```python
from build123d import *

# Parameters (mm, degrees)
SKETCH_1_W      = 27.85
SKETCH_1_H      = 27.85
SKETCH_1_R      = 1.25
SKETCH_1_R_2    = 6.5
EXTRUDE_1_DEPTH = 7
SKETCH_1_5_R    = 11
SKETCH_1_5_R_2  = 6.5
EXTRUDE_3_DEPTH = 9
CHAMFER_2_SIZE  = 0.4
CHAMFER_3_SIZE  = 0.2
FILLET_1_R      = 2


with BuildPart() as part:
    # Эскиз1 → Бобышка-Вытянуть1 (new body)
    with BuildSketch(Plane(origin=(0, 0, 0), x_dir=(1, 0, 0), z_dir=(0, 1, 0))):
        Rectangle(SKETCH_1_W, SKETCH_1_H)
        with Locations((-11.5, 11.5)):
            Circle(SKETCH_1_R, mode=Mode.SUBTRACT)
        with Locations((11.5, 11.5)):
            Circle(SKETCH_1_R, mode=Mode.SUBTRACT)
        with Locations((-11.5, -11.5)):
            Circle(SKETCH_1_R, mode=Mode.SUBTRACT)
        with Locations((11.5, -11.5)):
            Circle(SKETCH_1_R, mode=Mode.SUBTRACT)
        Circle(SKETCH_1_R_2, mode=Mode.SUBTRACT)
    extrude(amount=EXTRUDE_1_DEPTH)

    # Эскиз1<5> → Бобышка-Вытянуть3 (add)
    with BuildSketch(Plane(origin=(0, 0, 0), x_dir=(1, 0, 0), z_dir=(0, 1, 0))):
        Circle(SKETCH_1_5_R)
        Circle(SKETCH_1_5_R_2, mode=Mode.SUBTRACT)
    extrude(amount=EXTRUDE_3_DEPTH)

    # Фаска2
    chamfer_2_edges = [part.edges().sort_by_distance(p)[0] for p in [
        (-12.75, 7, 11.5),
        (10.25, 7, -11.5),
        (-12.75, 7, -11.5),
        (10.25, 7, 11.5),
    ]]
    chamfer(chamfer_2_edges, length=CHAMFER_2_SIZE)

    # Фаска3
    chamfer_3_edges = [part.edges().sort_by_distance(p)[0] for p in [
        (-6.5, 9, 0),
        (-11, 9, 0),
    ]]
    chamfer(chamfer_3_edges, length=CHAMFER_3_SIZE)

    # Скругление1
    fillet_1_edges = [part.edges().sort_by_distance(p)[0] for p in [
        (-13.925, 3.5, 13.925),
        (-13.925, 3.5, -13.925),
        (13.925, 3.5, -13.925),
        (13.925, 3.5, 13.925),
    ]]
    fillet(fillet_1_edges, radius=FILLET_1_R)


solid = part.part
```
Could you check a few things on this model? Use its own coordinates, in mm. A direction names the side the tool comes from. Give positions to 0.01 mm unless a question says otherwise; leave off trailing zeros. Order: outer loops, then holes, each group sorted by start corner. A loop starts at its lowest first (then second) coordinate and runs counter-clockwise, first axis right, second up.
Q1. If I drill on line 1 along Z through (x, y) = (11.5, 5) (3 decimals); line 2 along X through (y, z) = (6.75, 10.5) (3 decimals), over which ranges is the centre line in solid material (lowest first)?
Q2. We'd pull the mould along X, two halves only. Please class faces 1 (the flat face through (0, 3, -13.925)), 2 (the cylindrical face through (-13.355, 3.549, 13.324)), 3 (the cylindrical face through (10.579, 3.254, -12.345)): +X half, -X half, draft (parallel to the pull), parting line (faces both ways), or undercut.
Q3. I'm going to push flat-ended pins straight in: P1, Ø4, axis at x = 11.5, z = -11.5, coming from the -Y side; P2, Ø3, axis at x = 11.5, z = 11.5, coming from the +Y side. Where does each tip first touch, or does it pass through?
Q4. Suppose I cut it at B-B, the plane z = 0. Write out the boundary of the cut face in (x, y) (3 decimals).
Q5. Suppose I cut it at C-C, the plane y = 1.75. Write out the boundary of the cut face in (x, z) (3 decimals), and give its area (3 significant figures).
Q6. Suppose I cut it at A-A, the plane x = 0. Write out the boundary of the cut face in (y, z) (3 decimals), and give its area (3 significant figures).
Q7. Suppose I cut it at D-D, the plane z = -11.5. Write out the boundary of the cut face in (x, y) (3 decimals).
Q8. For faces 4 (the flat face through (-13.925, 3, 0)), 5 (the cylindrical face through (-2.38, 7.89, 10.74)), which set-ups out of +Z, -Z, +X, -X, +Y, -Y let a thin tool reach every point of the face, with its end or its side?
Solution:
1. line 1: z = -13.925 to -12.75, -10.25 to 10.25, 12.75 to 13.925
1. line 2: x = -13.925 to -12.48, -10.52 to 10.52, 12.48 to 13.925
2. face 1: draft
2. face 2: -X half
2. face 3: undercut
3. P1: stops at y = 0
3. P2: stops at y = 6.85
4. outline: (-13.925, 0) - (-6.5, 0) - (-6.5, 8.8) - (-6.7, 9) - (-10.8, 9) - (-11, 8.8) - (-11, 7) - (-13.925, 7) - close; (6.5, 0) - (13.925, 0) - (13.925, 7) - (11, 7) - (11, 8.8) - (10.8, 9) - (6.7, 9) - (6.5, 8.8) - close
5. outline: (-13.925, -11.925) arc R2 ccw to (-11.925, -13.925) - (11.925, -13.925) arc R2 ccw to (13.925, -11.925) - (13.925, 11.925) arc R2 ccw to (11.925, 13.925) - (-11.925, 13.925) arc R2 ccw to (-13.925, 11.925) - close; hole circle Ø2.5 at (-11.5, -11.5); hole circle Ø2.5 at (-11.5, 11.5); hole circle Ø13 at (0, 0); hole circle Ø2.5 at (11.5, -11.5); hole circle Ø2.5 at (11.5, 11.5)
5. area: 620 mm2
6. outline: (0, -13.925) - (7, -13.925) - (7, -11) - (8.8, -11) - (9, -10.8) - (9, -6.7) - (8.8, -6.5) - (0, -6.5) - close; (0, 6.5) - (8.8, 6.5) - (9, 6.7) - (9, 10.8) - (8.8, 11) - (7, 11) - (7, 13.925) - (0, 13.925) - close
6. area: 122 mm2
7. outline: (-13.925, 0) - (-12.75, 0) - (-12.75, 6.6) - (-13.15, 7) - (-13.925, 7) - close; (-10.25, 0) - (10.25, 0) - (10.25, 6.6) - (9.85, 7) - (-9.85, 7) - (-10.25, 6.6) - close; (12.75, 0) - (13.925, 0) - (13.925, 7) - (13.15, 7) - (12.75, 6.6) - close
8. face 4: +Z, -Z, -X, +Y, -Y
8. face 5: +Y
